Build history of the part. All positions in model axes, mm. A direction names the side the tool comes from. Round coordinates to 2 decimals unless told otherwise and drop trailing zeros. Order: outer loops, then holes, each group sorted by start corner. A loop starts at its lowest first (then second) coordinate and runs counter-clockwise, first axis right, second up. Notation, with made-up numbers: (66, 80.25) -> (93, 80.25) arc R7 ccw to (93, 85.25) -> close; hole circle Ø3 at (80.5, 4.5). An arc over 180 degrees is marked (long way). Answer as a JSON object with one key per item and string values.
from build123d import *

# Parameters (mm, degrees)
F0_R           = 10
F1_DEPTH       = 15
F2_D           = 10
F2_DEPTH       = 8
F2_TIP         = 3.0043030951
F6_D           = 2.5
F6_DEPTH       = 18
F6_START       = 0.5428599
F6_CBORE_D     = 6.5
F6_CBORE_DEPTH = 3
F6_TIP         = 0.7510757738


with BuildPart() as f1:
    # F0 (on Right) → F1 (new body)
    with BuildSketch(Plane.YZ):
        Circle(F0_R)
    extrude(amount=F1_DEPTH)

    # F2
    with Locations(Plane(origin=(0, 0, 0), x_dir=(0, 1, 0), z_dir=(-1, 0, 0))):
        with Locations((0, 0)):
            Hole(F2_D / 2, depth=F2_DEPTH)
            with Locations((0, 0, -(F2_DEPTH + F2_TIP / 2))):  # 118° drill point
                Cone(0, F2_D / 2, F2_TIP, mode=Mode.SUBTRACT)

    # F6
    # its depths count from where the whole tool has entered the part; down to there all is cleared
    with Locations(Plane.XY.offset(10).offset(-F6_START)):
        with Locations((5, 0)):
            CounterBoreHole(F6_D / 2, F6_CBORE_D / 2, F6_CBORE_DEPTH, depth=F6_DEPTH)
            with Locations((0, 0, -(F6_DEPTH + F6_TIP / 2))):  # 118° drill point
                Cone(0, F6_D / 2, F6_TIP, mode=Mode.SUBTRACT)


solid = f1.part
1) Cut at B-B, the plane x = 11.5. Give the cut face in (y, z), plus the area to 3 significant figures.
Checked values:
{"outline": "circle Ø20 at (0, 0)", "area": "314 mm²"}
2) Flat gauge pins, fed straight in: pin 1 Ø3 at (x, z) = (2.5, 5) entering from -Y; pin 2 Ø3 at (x, y) = (5, 0) entering from +Z; pin 3 Ø1.5 at (x, y) = (8.5, -8) entering from +Z. Where does each tip first touch, or does it go through?
Checked values:
{"pin 1": "stops at y = -9.37", "pin 2": "stops at z = 6.46", "pin 3": "stops at z = 6.89"}
3) Probe L1, parallel to X at y = 0, z = 6.05; L2, parallel to Z at x = 2.5, y = 0; L3, parallel to X at y = 0, z = 8.6. List the from-to ranges inside material, lowest first. Write a range as from..to.
Checked values:
{"L1": "x = 0..3.75, 6.25..15", "L2": "z = -10..-5, 5..6.46", "L3": "x = 0..1.75, 8.25..15"}
4) Cut at A-A, the plane z = 8.5. Give the cut face in (x, y), plus the area to 3 significant figures.
Checked values:
{"outline": "(0, -5.27) -> (15, -5.27) -> (15, 5.27) -> (0, 5.27) -> close; hole circle Ø6.5 at (5, 0)", "area": "125 mm²"}
5) Cut at C-C, the plane y = 5.5. Give the cut face in (x, z).
Checked values:
{"outline": "(0, -8.35) -> (15, -8.35) -> (15, 8.35) -> (0, 8.35) -> close"}
6) Which spindle directions (+Z, -Z, +X, -X, +Y, -Y) get a long thin tool onto all of the face, cutting with end or side? Do faces 4 (the face through (0, -5, -2)), 5 (the face through (3.81, 0.38, 5.64)), 6 (the face through (4.056, -2.307, 4.436)). Say none if no direction does.
Checked values:
{"face 4": "+Z, -Z, -X, +Y, -Y", "face 5": "+Z", "face 6": "-X"}
7) Pull direction Y, two halves, no side cores. Call faces 1 (the face through (7.4, -2.17, -9.76)), 2 (the face through (15, 0, 0)), 3 (the face through (6.4, 0, 6.457)): pulls with the +Y half, pulls with the -Y half, needs draft (parallel to the pull), parting line crosses it, or undercut.
Checked values:
{"face 1": "parting line crosses it", "face 2": "needs draft", "face 3": "undercut"}
